```python
from build123d import *

# Parameters (mm, degrees)
SKETCH1_W           = 40
SKETCH1_H           = 20
BOSS_EXTRUDE1_DEPTH = 36.5
SKETCH2_W           = 5
SKETCH2_H           = 2.4
BOSS_EXTRUDE2_DEPTH = 20
CUT_EXTRUDE1_DEPTH  = 44.881915409
BOSS_EXTRUDE3_DEPTH = 4.25
SKETCH9_R           = 2.5
BOSS_EXTRUDE4_DEPTH = 3
FILLET1_R           = 3
FILLET2_R           = 1


with BuildPart() as part:
    # Sketch1 → Boss-Extrude1 (new body)
    with BuildSketch(Plane.XY):
        Rectangle(SKETCH1_W, SKETCH1_H)
    extrude(amount=BOSS_EXTRUDE1_DEPTH)

    # Sketch2 → Boss-Extrude2 (add)
    with BuildSketch(Plane.XZ.offset(10)):
        with Locations((22.5, 33.45)):
            Rectangle(SKETCH2_W, SKETCH2_H)
        with Locations((-22.5, 33.45)):
            Rectangle(SKETCH2_W, SKETCH2_H)
    extrude(amount=-BOSS_EXTRUDE2_DEPTH)

    # Sketch3 → Cut-Extrude1 (cut, through all)
    with BuildSketch(Plane.XY.offset(34.65)):
        with BuildLine():
            Line((25, -0.55), (23.335164654, -0.55))
            ThreePointArc((23.335164654, -0.55), (21.5, 0), (23.335164654, 0.55))
            Line((23.335164654, 0.55), (25, 0.55))
            Line((25, 0.55), (25, -0.55))
        make_face()
        with BuildLine():
            Line((-25, 0.55), (-23.335164654, 0.55))
            ThreePointArc((-23.335164654, 0.55), (-21.5, 0), (-23.335164654, -0.55))
            Line((-23.335164654, -0.55), (-25, -0.55))
            Line((-25, -0.55), (-25, 0.55))
        make_face()
    extrude(amount=-CUT_EXTRUDE1_DEPTH, mode=Mode.SUBTRACT)

    # Sketch4 → Boss-Extrude3 (add)
    with BuildSketch(Plane.XY.offset(36.5)):
        with BuildLine():
            ThreePointArc((-7.632955955, 0.638410329), (-20, 0), (-7.632955955, -0.638410329))
            ThreePointArc((-7.632955955, -0.638410329), (-7.625027484, -0.596751111), (-7.610171977, -0.557031281))
            ThreePointArc((-7.610171977, -0.557031281), (-7.484785169, 0), (-7.610171977, 0.557031281))
            ThreePointArc((-7.610171977, 0.557031281), (-7.625027484, 0.596751111), (-7.632955955, 0.638410329))
        make_face()
    extrude(amount=BOSS_EXTRUDE3_DEPTH)

    # Sketch9 → Boss-Extrude4 (add)
    with BuildSketch(Plane.XY.offset(40.75)):
        with Locations((-13.8, 0)):
            Circle(SKETCH9_R)
    extrude(amount=BOSS_EXTRUDE4_DEPTH)

    # Fillet1
    fillet1_edges = [part.edges().sort_by_distance(p)[0] for p in [
        (0, -10, 0),
        (-20, 0, 0),
        (0, 10, 0),
        (20, 0, 0),
    ]]
    fillet(fillet1_edges, radius=FILLET1_R)

    # Fillet2
    fillet2_edges = [part.edges().sort_by_distance(p)[0] for p in [
        (0, -10, 36.5),
        (20, 0, 36.5),
        (0, 10, 36.5),
    ]]
    fillet(fillet2_edges, radius=FILLET2_R)


solid = part.part
```
The listing builds one solid part. Answer for the finished solid, in the listing's coordinates (mm). A direction names the side the tool comes from. Give positions to 0.01 mm unless a question says otherwise; leave off trailing zeros. Write each loop counter-clockwise with the first axis right and the second up, starting at its lowest first coordinate (ties: lowest second). Pieces come first, ordered by that corner, then holes. Notation, with made-up numbers: (61, 63) -> (66, 63) arc R13 ccw to (66, 87) -> close; hole circle Ø1 at (34, 42). An arc over 180 degrees is marked (long way). Write item = value, one per line. Start each with the question number.
1) Which of the six approach directions +Z, -Z, +X, -X, +Y, -Y give full straight-line access (tool end or side, diameter ignored) to faces 1 (the face through (20, 0, 17)), 2 (the face through (-24, -0.55, 33)), 3 (the face through (21, 0, 34.65)), 4 (the face through (24, -0.55, 33))?
2) The part is cut by section C-C, the plane z = 10. Determine the outline of the cut face in (x, y).
3) Determine the mould class of faces 5 (the face through (-21.5, 0, 33.5)), 6 (the face through (-20, 0, 17)), 7 (the face through (0.28, 9.14, 0.9)) for opening direction Y: +Y half, -Y half, draft (parallel to the pull), parting line (faces both ways), or undercut.
4) The part is cut by section A-A, the plane x = 22.5. Determine the outline of the cut face in (y, z).
5) The part is cut by section B-B, the plane x = -4.5. Determine the outline of the cut face in (y, z), and give its area (3 significant figures).
6) The part is cut by section D-D, the plane y = -4.75. Determine the outline of the cut face in (x, z).
7) Straight lines are drawn through the part: line 1 along Y through (x, z) = (22.5, 34.1); line 2 along X through (y, z) = (0, 32.8); line 3 along Z through (x, y) = (-12, -4). For each, find the intervals that lie inside material, in ascending order.
8) Each of these flat-tipped pins is pushed along its axis until it touches: pin 1 (1.5 mm diameter, centred on x = 22.5, y = 4.5, fed in from +Z); pin 2 (2 mm diameter, centred on x = -19, y = 0.5, fed in from -Z); pin 3 (4 mm diameter, centred on x = -23.5, y = -5, fed in from -Z). Where does it stop, or does it pass through?
Solutions:
q1.face_1 = -Z, +X, +Y, -Y
q1.face_2 = +Z, -Z, -X
q1.face_3 = +Z, +X, +Y, -Y
q1.face_4 = +Z, -Z, +X
q2.outline = (-20, -10) -> (20, -10) -> (20, 10) -> (-20, 10) -> close
q3.face_5 = undercut
q3.face_6 = draft
q3.face_7 = +Y half
q4.outline = (-10, 32.25) -> (-1, 32.25) -> (-1, 34.65) -> (-10, 34.65) -> close; (1, 32.25) -> (10, 32.25) -> (10, 34.65) -> (1, 34.65) -> close
q5.outline = (-10, 3) arc R3 ccw to (-7, 0) -> (7, 0) arc R3 ccw to (10, 3) -> (10, 35.5) arc R1 ccw to (9, 36.5) -> (-9, 36.5) arc R1 ccw to (-10, 35.5) -> close
q5.area = 726 mm²
q6.outline = (-25, 32.25) -> (-20, 32.25) -> (-20, 3) arc R3 ccw to (-17, 0) -> (17, 0) arc R3 ccw to (20, 3) -> (20, 32.25) -> (25, 32.25) -> (25, 34.65) -> (20, 34.65) -> (20, 35.5) arc R1 ccw to (19, 36.5) -> (-9.82, 36.5) -> (-9.82, 40.75) -> (-17.78, 40.75) -> (-17.78, 36.5) -> (-20, 36.5) -> (-20, 34.65) -> (-25, 34.65) -> close
q7.line_1 = -10 to -1, 1 to 10
q7.line_2 = -21.5 to 21.5
q7.line_3 = 0 to 40.75
q8.pin_1 = 34.65
q8.pin_2 = 0.17
q8.pin_3 = 32.25
